```python
from build123d import *

# Parameters (mm, degrees)
CROQUIS1_R              = 1.5
CROQUIS1_R_2            = 20
SALIENTE_EXTRUIR1_DEPTH = 5


with BuildPart() as part:
    # Croquis1 → Saliente-Extruir1 (new body)
    with BuildSketch(Plane.XY):
        with BuildLine():
            Line((0, 0), (5, 0))
            Line((5, 0), (5, 5))
            Line((5, 5), (9.25, 5))
            Line((9.25, 5), (9.25, 14))
            Line((9.25, 14), (5.75, 14))
            Line((5.75, 14), (5.75, 17))
            Line((5.75, 17), (9.25, 17))
            Line((9.25, 17), (9.25, 20))
            Line((9.25, 20), (12.25, 20))
            Line((12.25, 20), (12.25, 17))
            Line((12.25, 17), (15.75, 17))
            Line((15.75, 17), (15.75, 14))
            Line((15.75, 14), (12.25, 14))
            Line((12.25, 14), (12.25, 5))
            Line((12.25, 5), (21.5, 5))
            Line((21.5, 5), (21.5, 11.24))
            ThreePointArc((21.5, 11.24), (25, 14.74), (28.5, 11.24))
            Line((28.5, 11.24), (28.5, 5))
            Line((28.5, 5), (37.75, 5))
            Line((37.75, 5), (37.75, 14))
            Line((37.75, 14), (34.25, 14))
            Line((34.25, 14), (34.25, 17))
            Line((34.25, 17), (37.75, 17))
            Line((37.75, 17), (37.75, 20))
            Line((37.75, 20), (40.75, 20))
            Line((40.75, 20), (40.75, 17))
            Line((40.75, 17), (44.25, 17))
            Line((44.25, 17), (44.25, 14))
            Line((44.25, 14), (40.75, 14))
            Line((40.75, 14), (40.75, 5))
            Line((40.75, 5), (45, 5))
            Line((45, 5), (45, 0))
            Line((45, 0), (50, 0))
            Line((50, 0), (50, 77.5))
            Line((50, 77.5), (40, 77.5))
            Line((40, 77.5), (40, 82.5))
            Line((40, 82.5), (10, 82.5))
            Line((10, 82.5), (10, 77.5))
            Line((10, 77.5), (0, 77.5))
            Line((0, 77.5), (0, 0))
        make_face()
        with Locations((25, 80)):
            Circle(CROQUIS1_R, mode=Mode.SUBTRACT)
        with Locations((25, 52.5)):
            Circle(CROQUIS1_R_2, mode=Mode.SUBTRACT)
    extrude(amount=SALIENTE_EXTRUIR1_DEPTH)


solid = part.part
```
Design review of the part built by this model. Coordinates are the model's own, in mm. A direction names the side the tool comes from. Coordinates: 2 decimals unless noted, no trailing zeros. Order: outer loops, then holes, each group sorted by start corner. A loop starts at its lowest first (then second) coordinate and runs counter-clockwise, first axis right, second up.
1) Take a section at D-D, the plane z = 3.25. State how many separate pieces and enclosed holes the cut face has, and give its area (3 significant figures).
2) Clearance check with flat-ended pins moving along their axes: pin 1 (3 mm diameter, centred on x = 8, z = 3, fed in from +Y); pin 2 (1.8 mm diameter, centred on x = 15, z = 3, fed in from -Y); pin 3 (0.9 mm diameter, centred on x = 11.5, z = 3, fed in from -Y). State where each tip first meets the part, or that it passes through.
3) For faces 1 (the flat face through (36, 14, 2)), 2 (the flat face through (45, 77.5, 2)), 3 (the flat face through (11, 20, 2)), list the 3-axis set-ups (+Z, -Z, +X, -X, +Y, -Y) from which the entire face can be reached by the end or side of a thin tool; tool diameter is ignored.
4) Mouldability with a two-part tool opening along Y and no side actions: class faces 4 (the cylindrical face through (24.92, 14.74, 2.46)), 5 (the flat face through (28.5, 8, 2)), 6 (the flat face through (42, 17, 2)) as +Y half, -Y half, draft (parallel to the pull), parting line (faces both ways), or undercut.
5) Wall thickness on line 1 along Y through (x, z) = (25, 1.4); line 2 along X through (y, z) = (7.5, 2.85); line 3 along X through (y, z) = (80, 2.05): over which ranges is each line inside the solid? List them lowest first.
6) Take a section at B-B, the plane x = 25. Give the boundary of the cut face in (y, z).
7) Take a section at C-C, the plane x = 31.5. Give the boundary of the cut face in (y, z).
8) Take a section at A-A, the plane y = 52.5. Give the boundary of the cut face in (x, z).
Returned:
1. separate pieces: 1
1. enclosed holes: 2
1. area: 2,370 mm2
2. pin 1: stops at y = 77.5
2. pin 2: stops at y = 5
2. pin 3: stops at y = 20
3. face 1: +Z, -Z
3. face 2: +Z, -Z, +X, +Y
3. face 3: +Z, -Z, -Y
4. face 4: -Y half
4. face 5: draft
4. face 6: undercut
5. line 1: y = 14.74 to 32.5, 72.5 to 78.5, 81.5 to 82.5
5. line 2: x = 0 to 9.25, 12.25 to 21.5, 28.5 to 37.75, 40.75 to 50
5. line 3: x = 10 to 23.5, 26.5 to 40
6. outline: (14.74, 0) - (32.5, 0) - (32.5, 5) - (14.74, 5) - close; (72.5, 0) - (78.5, 0) - (78.5, 5) - (72.5, 5) - close; (81.5, 0) - (82.5, 0) - (82.5, 5) - (81.5, 5) - close
7. outline: (5, 0) - (33.59, 0) - (33.59, 5) - (5, 5) - close; (71.41, 0) - (82.5, 0) - (82.5, 5) - (71.41, 5) - close
8. outline: (0, 0) - (5, 0) - (5, 5) - (0, 5) - close; (45, 0) - (50, 0) - (50, 5) - (45, 5) - close
